from build123d import *

# Parameters (mm, degrees)
ESQUISSE1_W                = 30
ESQUISSE1_H                = 300
BOSS_EXTRU_1_DEPTH         = 10
ESQUISSE2_W                = 10
ESQUISSE2_H                = 10
ENL_V_MAT_EXTRU_1_DEPTH    = 10
R_P_TITION_LIN_AIRE1_COUNT = 4
R_P_TITION_LIN_AIRE1_PITCH = 20
ENL_V_MAT_EXTRU_2_DEPTH    = 10


with BuildPart() as part:
    # Esquisse1 → Boss.-Extru.1 (new body)
    with BuildSketch(Plane.XY):
        with Locations((-15, 150)):
            Rectangle(ESQUISSE1_W, ESQUISSE1_H)
    extrude(amount=BOSS_EXTRU_1_DEPTH)

    # Esquisse2 → Enlèv. mat.-Extru.1 (cut)
    with BuildSketch(Plane.XY.offset(10)):
        with Locations((-25, 162)):
            Rectangle(ESQUISSE2_W, ESQUISSE2_H)
    enl_v_mat_extru_1 = extrude(amount=-ENL_V_MAT_EXTRU_1_DEPTH, mode=Mode.SUBTRACT)

    # Répétition linéaire1: Enlèv. mat.-Extru.1 ×4
    with Locations(*[(0, -i * R_P_TITION_LIN_AIRE1_PITCH, 0) for i in range(1, R_P_TITION_LIN_AIRE1_COUNT)]):
        add(enl_v_mat_extru_1, mode=Mode.SUBTRACT)

    # Esquisse3 → Enlèv. mat.-Extru.2 (cut)
    with BuildSketch(Plane.XY.offset(10)):
        with BuildLine():
            Line((-4, 171), (-4, 221))
            ThreePointArc((-4, 221), (-10, 227), (-16, 221))
            Line((-16, 221), (-16, 171))
            ThreePointArc((-16, 171), (-10, 165), (-4, 171))
        make_face()
    extrude(amount=-ENL_V_MAT_EXTRU_2_DEPTH, mode=Mode.SUBTRACT)


solid = part.part
Geometry check sheet. Reference: the model listing, model coordinates, mm. A direction names the side the tool comes from. Give positions to 0.01 mm unless a question says otherwise; leave off trailing zeros. Write each loop counter-clockwise with the first axis right and the second up, starting at its lowest first coordinate (ties: lowest second). Pieces come first, ordered by that corner, then holes.
1) Cross-section at B-B (z = 8.5). Record the boundary of the cut face in (x, y).
Values follow:
outline: (-30, 0) - (0, 0) - (0, 300) - (-30, 300) - (-30, 167) - (-20, 167) - (-20, 157) - (-30, 157) - (-30, 147) - (-20, 147) - (-20, 137) - (-30, 137) - (-30, 127) - (-20, 127) - (-20, 117) - (-30, 117) - (-30, 107) - (-20, 107) - (-20, 97) - (-30, 97) - close; hole (-16, 171) arc R6 ccw to (-4, 171) - (-4, 221) arc R6 ccw to (-16, 221) - close
2) Thickness scan on line 1 (Y direction, x = -28.5, z = 3); line 2 (X direction, y = 185, z = 2.25); line 3 (Y direction, x = -14.5, z = 5). Record the ranges inside material, lowest first.
Values follow:
line 1: y = 0 to 97, 107 to 117, 127 to 137, 147 to 157, 167 to 300
line 2: x = -30 to -16, -4 to 0
line 3: y = 0 to 167.03, 224.97 to 300
3) Release check for a two-part mould opening along Y. For faces 1 (the face through (-20, 122, 5)), 2 (the face through (-30, 132, 5)), 3 (the face through (-15, 300, 5)) record: released by +Y, released by -Y, zero draft, split by the parting line, or undercut.
Values follow:
face 1: undercut
face 2: zero draft
face 3: released by +Y
4) Set-up check for faces 4 (the face through (-25, 97, 5)), 5 (the face through (-10, 227, 5)), 6 (the face through (-30, 152, 5)): record each of +Z, -Z, +X, -X, +Y, -Y from which the full face is reachable in a straight line by a thin tool's end or side.
Values follow:
face 4: +Z, -Z, -X
face 5: +Z, -Z
face 6: +Z, -Z, -X, +Y, -Y
5) Go/stop test with a flat-tipped pin: pin 1 Ø5 at (y, z) = (160, 4) entering from -X. Record where the tip stops, or that it passes through.
Values follow:
pin 1: stops at x = -20
6) Cross-section at C-C (y = 123.5). Record the boundary of the cut face in (x, z), plus the area to 3 significant figures.
Values follow:
outline: (-20, 0) - (0, 0) - (0, 10) - (-20, 10) - close
area: 200 mm2
7) Cross-section at A-A (x = -10). Record the boundary of the cut face in (y, z), plus the area to 3 significant figures.
Values follow:
outline: (0, 0) - (165, 0) - (165, 10) - (0, 10) - close; (227, 0) - (300, 0) - (300, 10) - (227, 10) - close
area: 2,380 mm2
